Work out the finished part from the listing and answer in its coordinate system (mm). A direction names the side the tool comes from. Round coordinates to 2 decimals unless told otherwise and drop trailing zeros. Write each loop counter-clockwise with the first axis right and the second up, starting at its lowest first coordinate (ties: lowest second). Pieces come first, ordered by that corner, then holes. Notation, with made-up numbers: (55.25, 48.5) - (71.25, 48.5) arc R12 cw to (71.25, 58.5) - close; hole circle Ø6 at (43.5, 0.5). An arc over 180 degrees is marked (long way). Answer as a JSON object with one key per item and string values.
```python
from build123d import *

# Parameters (mm, degrees)
SKETCH1_R               = 11
SKETCH1_R_2             = 16.5
SKETCH1_R_3             = 1.25
SKETCH1_R_4             = 1.5
SKETCH1_R_5             = 1.8
BOSS_EXTRUDE1_DEPTH     = 6
FILLET1_R               = 10
SKETCH2_W               = 15
SKETCH2_H               = 22
BOSS_EXTRUDE2_DEPTH     = 6
CHAMFER1_SIZE           = 1
SKETCH3_R               = 1
CUT_EXTRUDE1_DEPTH      = 159.031622895
MOVE_FACE1_OUTLINE_R    = 11
MOVE_FACE1_OUTLINE_R_2  = 10.92
MOVE_FACE1_OUTLINE_R_3  = 16.5
MOVE_FACE1_OUTLINE_R_4  = 16.42
MOVE_FACE1_OUTLINE_R_5  = 1.25
MOVE_FACE1_OUTLINE_R_6  = 1.17
MOVE_FACE1_OUTLINE_R_7  = 1.5
MOVE_FACE1_OUTLINE_R_8  = 1.42
MOVE_FACE1_OUTLINE_R_9  = 1.8
MOVE_FACE1_OUTLINE_R_10 = 1.72
MOVE_FACE1_DEPTH        = 6


# Read off the part's stored shape, not the designer's step: Move Face1
with BuildPart() as part:
    # Sketch1 → Boss-Extrude1 (new body)
    with BuildSketch(Plane.XY):
        with BuildLine():
            Line((-40.498784978, 0), (0, 0))
            Line((0, 0), (0, 75))
            ThreePointArc((0, 75), (-37.5, 112.5), (-75, 75))
            Line((-75, 75), (-75, 55))
            Line((-75, 55), (-83.323029145, 55))
            ThreePointArc((-83.323029145, 55), (-110.823029145, 27.5), (-83.323029145, 0))
            Line((-83.323029145, 0), (-40.498784978, 0))
        make_face()
        with Locations((-83.323029145, 27.5)):
            Circle(SKETCH1_R, mode=Mode.SUBTRACT)
        with Locations((-37.5, 75)):
            Circle(SKETCH1_R_2, mode=Mode.SUBTRACT)
        with Locations((-83.323029145, 50.5)):
            Circle(SKETCH1_R_3, mode=Mode.SUBTRACT)
        with Locations((-67.059573177, 43.763455967)):
            Circle(SKETCH1_R_4, mode=Mode.SUBTRACT)
        with Locations((-60.323029145, 27.5)):
            Circle(SKETCH1_R_3, mode=Mode.SUBTRACT)
        with Locations((-67.059573177, 11.236544033)):
            Circle(SKETCH1_R_4, mode=Mode.SUBTRACT)
        with Locations((-83.323029145, 4.5)):
            Circle(SKETCH1_R_3, mode=Mode.SUBTRACT)
        with Locations((-37.5, 102.5)):
            Circle(SKETCH1_R_5, mode=Mode.SUBTRACT)
        with Locations((-10, 75)):
            Circle(SKETCH1_R_5, mode=Mode.SUBTRACT)
        with Locations((-37.5, 47.5)):
            Circle(SKETCH1_R_5, mode=Mode.SUBTRACT)
        with Locations((-65, 75)):
            Circle(SKETCH1_R_5, mode=Mode.SUBTRACT)
        with Locations((-18.054563517, 94.445436483)):
            Circle(SKETCH1_R_4, mode=Mode.SUBTRACT)
        with Locations((-18.054563517, 55.554563517)):
            Circle(SKETCH1_R_4, mode=Mode.SUBTRACT)
        with Locations((-56.945436483, 55.554563517)):
            Circle(SKETCH1_R_4, mode=Mode.SUBTRACT)
        with Locations((-56.945436483, 94.445436483)):
            Circle(SKETCH1_R_4, mode=Mode.SUBTRACT)
    extrude(amount=BOSS_EXTRUDE1_DEPTH)

    # Fillet1
    fillet1_edges = [part.edges().sort_by_distance(p)[0] for p in [
        (-75, 55, 3),
    ]]
    fillet(fillet1_edges, radius=FILLET1_R)

    # Sketch2 → Boss-Extrude2 (add)
    with BuildSketch(Plane(origin=(0, 0, 0), x_dir=(-1, 0, 0), z_dir=(0, 0, -1))):
        with Locations((7.5, -11)):
            Rectangle(SKETCH2_W, SKETCH2_H)
        with Locations((37.5, -11)):
            Rectangle(SKETCH2_W, SKETCH2_H)
        with Locations((67.5, -11)):
            Rectangle(SKETCH2_W, SKETCH2_H)
    extrude(amount=-BOSS_EXTRUDE2_DEPTH)

    # Chamfer1
    chamfer1_edges = [part.edges().sort_by_distance(p)[0] for p in [
        (-30, -22, 3),
        (-45, -22, 3),
        (-60, -22, 3),
        (-75, -22, 3),
        (0, -22, 3),
        (-15, -22, 3),
    ]]
    chamfer(chamfer1_edges, length=CHAMFER1_SIZE)

    # Sketch3 → Cut-Extrude1 (cut, through all)
    with BuildSketch(Plane.XY.offset(6)):
        with Locations((-75, 0)):
            Circle(SKETCH3_R)
        with Locations((-60, 0)):
            Circle(SKETCH3_R)
        with Locations((-45, 0)):
            Circle(SKETCH3_R)
        with Locations((-30, 0)):
            Circle(SKETCH3_R)
        with Locations((-15, 0)):
            Circle(SKETCH3_R)
    extrude(amount=-CUT_EXTRUDE1_DEPTH, mode=Mode.SUBTRACT)

    # Move Face1 outline → Move Face1 (add)
    # profile 1 of 20: a face of its own
    with BuildSketch(Plane.XY):
        with BuildLine():
            Line((-59.003205136, -0.08), (-45.996794864, -0.08))
            ThreePointArc((-45.996794864, -0.08), (-45.999198395, -0.04003209), (-46, 0))
            Line((-46, 0), (-59, 0))
            ThreePointArc((-59, 0), (-59.000801605, -0.04003209), (-59.003205136, -0.08))
        make_face()
    # profile 2 of 20: a face of its own
    with BuildSketch(Plane.XY):
        with BuildLine():
            Line((-45, -21), (-45, -1))
            ThreePointArc((-45, -1), (-45.04003209, -0.999198395), (-45.08, -0.996794864))
            Line((-45.08, -0.996794864), (-45.08, -21.033137085))
            Line((-45.08, -21.033137085), (-44.033137085, -22.08))
            Line((-44.033137085, -22.08), (-30.966862915, -22.08))
            Line((-30.966862915, -22.08), (-29.92, -21.033137085))
            Line((-29.92, -21.033137085), (-29.92, -0.996794864))
            ThreePointArc((-29.92, -0.996794864), (-29.95996791, -0.999198395), (-30, -1))
            Line((-30, -1), (-30, -21))
            Line((-30, -21), (-31, -22))
            Line((-31, -22), (-44, -22))
            Line((-44, -22), (-45, -21))
        make_face()
    # profile 3 of 20: a face of its own
    with BuildSketch(Plane.XY):
        with BuildLine():
            ThreePointArc((-59.92, -0.996794864), (-59.95996791, -0.999198395), (-60, -1))
            Line((-60, -1), (-60, -21))
            Line((-60, -21), (-61, -22))
            Line((-61, -22), (-74, -22))
            Line((-74, -22), (-75, -21))
            Line((-75, -21), (-75, -1))
            ThreePointArc((-75, -1), (-75.04003209, -0.999198395), (-75.08, -0.996794864))
            Line((-75.08, -0.996794864), (-75.08, -21.033137085))
            Line((-75.08, -21.033137085), (-74.033137085, -22.08))
            Line((-74.033137085, -22.08), (-60.966862915, -22.08))
            Line((-60.966862915, -22.08), (-59.92, -21.033137085))
            Line((-59.92, -21.033137085), (-59.92, -0.996794864))
        make_face()
    # profile 4 of 20: a face of its own
    with BuildSketch(Plane.XY):
        with BuildLine():
            Line((-16, 0), (-29, 0))
            ThreePointArc((-29, 0), (-29.000801605, -0.04003209), (-29.003205136, -0.08))
            Line((-29.003205136, -0.08), (-15.996794864, -0.08))
            ThreePointArc((-15.996794864, -0.08), (-15.999198395, -0.04003209), (-16, 0))
        make_face()
    # profile 5 of 20: a face of its own
    with BuildSketch(Plane.XY):
        with BuildLine():
            ThreePointArc((-75.996794864, -0.08), (-75.999198395, -0.04003209), (-76, 0))
            Line((-76, 0), (-83.323029145, 0))
            ThreePointArc((-83.323029145, 0), (-110.816150501, 26.884956844), (-84.552807772, 54.972488867))
            ThreePointArc((-84.552807772, 54.972488867), (-77.772555006, 58.051331596), (-75, 64.962484818))
            Line((-75, 64.962484818), (-75, 75))
            ThreePointArc((-75, 75), (-37.5, 112.5), (0, 75))
            Line((0, 75), (0, -21))
            Line((0, -21), (-1, -22))
            Line((-1, -22), (-14, -22))
            Line((-14, -22), (-15, -21))
            Line((-15, -21), (-15, -1))
            ThreePointArc((-15, -1), (-15.04003209, -0.999198395), (-15.08, -0.996794864))
            Line((-15.08, -0.996794864), (-15.08, -21.033137085))
            Line((-15.08, -21.033137085), (-14.033137085, -22.08))
            Line((-14.033137085, -22.08), (-0.966862915, -22.08))
            Line((-0.966862915, -22.08), (0.08, -21.033137085))
            Line((0.08, -21.033137085), (0.08, 75))
            ThreePointArc((0.08, 75), (-37.5, 112.58), (-75.08, 75))
            Line((-75.08, 75), (-75.08, 64.962484818))
            ThreePointArc((-75.08, 64.962484818), (-77.830374566, 58.106620822), (-84.55638531, 55.052408834))
            ThreePointArc((-84.55638531, 55.052408834), (-110.896130491, 26.883167628), (-83.323029145, -0.08))
            Line((-83.323029145, -0.08), (-75.996794864, -0.08))
        make_face()
    # profile 6 of 20: a face of its own
    with BuildSketch(Plane.XY):
        with Locations((-83.323029145, 27.5)):
            Circle(MOVE_FACE1_OUTLINE_R)
        with Locations((-83.323029145, 27.5)):
            Circle(MOVE_FACE1_OUTLINE_R_2, mode=Mode.SUBTRACT)
    # profile 7 of 20: a face of its own
    with BuildSketch(Plane.XY):
        with Locations((-37.5, 75)):
            Circle(MOVE_FACE1_OUTLINE_R_3)
        with Locations((-37.5, 75)):
            Circle(MOVE_FACE1_OUTLINE_R_4, mode=Mode.SUBTRACT)
    # profile 8 of 20: a face of its own
    with BuildSketch(Plane.XY):
        with Locations((-83.323029145, 50.5)):
            Circle(MOVE_FACE1_OUTLINE_R_5)
        with Locations((-83.323029145, 50.5)):
            Circle(MOVE_FACE1_OUTLINE_R_6, mode=Mode.SUBTRACT)
    # profile 9 of 20: a face of its own
    with BuildSketch(Plane.XY):
        with Locations((-67.059573177, 43.763455967)):
            Circle(MOVE_FACE1_OUTLINE_R_7)
        with Locations((-67.059573177, 43.763455967)):
            Circle(MOVE_FACE1_OUTLINE_R_8, mode=Mode.SUBTRACT)
    # profile 10 of 20: a face of its own
    with BuildSketch(Plane.XY):
        with Locations((-37.5, 102.5)):
            Circle(MOVE_FACE1_OUTLINE_R_9)
        with Locations((-37.5, 102.5)):
            Circle(MOVE_FACE1_OUTLINE_R_10, mode=Mode.SUBTRACT)
    # profile 11 of 20: a face of its own
    with BuildSketch(Plane.XY):
        with Locations((-60.323029145, 27.5)):
            Circle(MOVE_FACE1_OUTLINE_R_5)
        with Locations((-60.323029145, 27.5)):
            Circle(MOVE_FACE1_OUTLINE_R_6, mode=Mode.SUBTRACT)
    # profile 12 of 20: a face of its own
    with BuildSketch(Plane.XY):
        with Locations((-67.059573177, 11.236544033)):
            Circle(MOVE_FACE1_OUTLINE_R_7)
        with Locations((-67.059573177, 11.236544033)):
            Circle(MOVE_FACE1_OUTLINE_R_8, mode=Mode.SUBTRACT)
    # profile 13 of 20: a face of its own
    with BuildSketch(Plane.XY):
        with Locations((-83.323029145, 4.5)):
            Circle(MOVE_FACE1_OUTLINE_R_5)
        with Locations((-83.323029145, 4.5)):
            Circle(MOVE_FACE1_OUTLINE_R_6, mode=Mode.SUBTRACT)
    # profile 14 of 20: a face of its own
    with BuildSketch(Plane.XY):
        with Locations((-10, 75)):
            Circle(MOVE_FACE1_OUTLINE_R_9)
        with Locations((-10, 75)):
            Circle(MOVE_FACE1_OUTLINE_R_10, mode=Mode.SUBTRACT)
    # profile 15 of 20: a face of its own
    with BuildSketch(Plane.XY):
        with Locations((-37.5, 47.5)):
            Circle(MOVE_FACE1_OUTLINE_R_9)
        with Locations((-37.5, 47.5)):
            Circle(MOVE_FACE1_OUTLINE_R_10, mode=Mode.SUBTRACT)
    # profile 16 of 20: a face of its own
    with BuildSketch(Plane.XY):
        with Locations((-65, 75)):
            Circle(MOVE_FACE1_OUTLINE_R_9)
        with Locations((-65, 75)):
            Circle(MOVE_FACE1_OUTLINE_R_10, mode=Mode.SUBTRACT)
    # profile 17 of 20: a face of its own
    with BuildSketch(Plane.XY):
        with Locations((-18.054563517, 94.445436483)):
            Circle(MOVE_FACE1_OUTLINE_R_7)
        with Locations((-18.054563517, 94.445436483)):
            Circle(MOVE_FACE1_OUTLINE_R_8, mode=Mode.SUBTRACT)
    # profile 18 of 20: a face of its own
    with BuildSketch(Plane.XY):
        with Locations((-18.054563517, 55.554563517)):
            Circle(MOVE_FACE1_OUTLINE_R_7)
        with Locations((-18.054563517, 55.554563517)):
            Circle(MOVE_FACE1_OUTLINE_R_8, mode=Mode.SUBTRACT)
    # profile 19 of 20: a face of its own
    with BuildSketch(Plane.XY):
        with Locations((-56.945436483, 55.554563517)):
            Circle(MOVE_FACE1_OUTLINE_R_7)
        with Locations((-56.945436483, 55.554563517)):
            Circle(MOVE_FACE1_OUTLINE_R_8, mode=Mode.SUBTRACT)
    # profile 20 of 20: a face of its own
    with BuildSketch(Plane.XY):
        with Locations((-56.945436483, 94.445436483)):
            Circle(MOVE_FACE1_OUTLINE_R_7)
        with Locations((-56.945436483, 94.445436483)):
            Circle(MOVE_FACE1_OUTLINE_R_8, mode=Mode.SUBTRACT)
    extrude(amount=MOVE_FACE1_DEPTH)


solid = part.part
```
Item 1: For faces 4 (the flat face through (-75.08, -11, 3)), 5 (the flat face through (-44, 46, 0)), 6 (the flat face through (-59.92, -11, 3)), determine the directions among +Z, -Z, +X, -X, +Y, -Y from which every point of the face is accessible in a straight line to the end or side of a thin tool.
Results found:
{"face 4": "+Z, -Z, -X, -Y", "face 5": "-Z, +X, -X, +Y, -Y", "face 6": "+Z, -Z, -Y"}
Item 2: A cutting plane is placed at B-B (y = -11.5). Write down the section's boundary in (x, z), and give its area (3 significant figures).
Results found:
{"outline": "(-75.08, 0) - (-59.92, 0) - (-59.92, 6) - (-75.08, 6) - close; (-45.08, 0) - (-29.92, 0) - (-29.92, 6) - (-45.08, 6) - close; (-15.08, 0) - (0.08, 0) - (0.08, 6) - (-15.08, 6) - close", "area": "273 mm²"}
Item 3: Determine the mould class of faces 1 (the cylindrical face through (-110.903, 27.481, 2.958)), 2 (the cylindrical face through (-10.37, 73.32, 2.96)), 3 (the flat face through (-29.92, -11, 3)) for opening direction Y: pulls with the +Y half, pulls with the -Y half, needs draft (parallel to the pull), parting line crosses it, or undercut.
Results found:
{"face 1": "parting line crosses it", "face 2": "undercut", "face 3": "needs draft"}
Item 4: Consider line 1 along Y through (x, z) = (-37.5, 1.35); line 2 along X through (y, z) = (-11, 4.9); line 3 along Y through (x, z) = (-45, 3.2). Determine where each line is inside the solid, lowest interval first.
Results found:
{"line 1": "-22.08 to 45.78, 49.22 to 58.58, 91.42 to 100.78, 104.22 to 112.58", "line 2": "-75.08 to -59.92, -45.08 to -29.92, -15.08 to 0.08", "line 3": "-21.11 to -1, 1 to 60.39, 89.61 to 111.82"}
Item 5: Each of these flat-tipped pins is pushed along its axis until it touches: P1, Ø1.8, axis at x = -51, z = 3, coming from the -Y side; P2, Ø1.7, axis at x = -67.06, y = 43.76, coming from the -Z side; P3, Ø2, axis at x = -78, z = 5, coming from the +Y side; P4, Ø2.5, axis at x = -75, y = 0, coming from the -Z side. Where does it stop, or does it pass through?
Results found:
{"P1": "y = -0.08", "P2": "through", "P3": "y = 59.1", "P4": "z = 0"}
Item 6: A cutting plane is placed at C-C (y = 102.5). Write down the section's boundary in (x, z), and give its area (3 significant figures).
Results found:
{"outline": "(-63.11, 0) - (-39.22, 0) - (-39.22, 6) - (-63.11, 6) - close; (-35.78, 0) - (-11.89, 0) - (-11.89, 6) - (-35.78, 6) - close", "area": "287 mm²"}
Item 7: A cutting plane is placed at A-A (x = -37.5). Write down the section's boundary in (y, z).
Results found:
{"outline": "(-22.08, 0) - (45.78, 0) - (45.78, 6) - (-22.08, 6) - close; (49.22, 0) - (58.58, 0) - (58.58, 6) - (49.22, 6) - close; (91.42, 0) - (100.78, 0) - (100.78, 6) - (91.42, 6) - close; (104.22, 0) - (112.58, 0) - (112.58, 6) - (104.22, 6) - close"}
Item 8: A cutting plane is placed at D-D (x = -80). Write down the section's boundary in (y, z).
Results found:
{"outline": "(-0.08, 0) - (17.1, 0) - (17.1, 6) - (-0.08, 6) - close; (37.9, 0) - (56.39, 0) - (56.39, 6) - (37.9, 6) - close"}
